from build123d import *

# Parameters (mm, degrees)
F0_W     = 76.2
F0_H     = 38.1
F1_DEPTH = 25.4
F2_R     = 3.175
F3_DEPTH = 25.4
F4_R     = 11.153796
F5_DEPTH = 38.1
F6_W     = 14.986
F6_H     = 12.7
F8_R     = 1.524


with BuildPart() as f1:
    # F0 (on Top) → F1 (new body)
    with BuildSketch(Plane.XY):
        with Locations((0.211801, -8.619163)):
            Rectangle(F0_W, F0_H)
    extrude(amount=F1_DEPTH)

    # F2 (on Top) → F3 (cut)
    with BuildSketch(Plane.XY):
        with Locations((-30.268199, 2.810837)):
            Circle(F2_R)
        with Locations((-30.268199, -20.049163)):
            Circle(F2_R)
        with Locations((30.691801, 2.810837)):
            Circle(F2_R)
        with Locations((30.691801, -20.049163)):
            Circle(F2_R)
    extrude(amount=F3_DEPTH, mode=Mode.SUBTRACT)

    # F4 (on face) → F5 (join)
    with BuildSketch(Plane.XY.offset(25.4)):
        with Locations((0, -7.839597)):
            Circle(F4_R)
    extrude(amount=F5_DEPTH)

    # F6 (on Front) → F7 (revolve, cut)
    with BuildSketch(Plane.XZ):
        with Locations((-11.421585, 44.041961)):
            Rectangle(F6_W, F6_H)
    revolve(axis=Axis((0, -7.839597, 63.5), (0, 0, 1)), mode=Mode.SUBTRACT)

    # F8
    f8_edges = [f1.edges().sort_by_distance(p)[0] for p in [
        (0.211801, -27.669163, 25.4),
        (-37.888199, -8.619163, 25.4),
        (0.211801, 10.430837, 25.4),
        (38.311801, -8.619163, 25.4),
    ]]
    fillet(f8_edges, radius=F8_R)


solid = f1.part
Check sheet for the modelled part. Datum: model origin and axes. Units: mm. A direction names the side the tool comes from. Coordinates: 2 decimals unless noted, no trailing zeros. Loops run counter-clockwise (first coordinate to the right, second up) from the corner with the lowest first, then second, coordinate; pieces in that order, holes last. Notation, with made-up numbers: (29, 61.25) -> (48, 61.25) arc R28 cw to (48, 94.25) -> close; hole circle Ø3 at (9.5, 89). An arc over 180 degrees is marked (long way). Write item = value, one per line. Start each with the question number.
1. Draft check along Z on faces 4 (the cylindrical face through (27.52, 2.95, 12.52)), 5 (the flat face through (0, -8, 0)), 6 (the flat face through (-2, 1, 37.692)). Enter one of: released by +Z, released by -Z, zero draft, split by the parting line, or undercut.
2. Section check C-C on x = 18.5. Record the cut outline in (y, z).
3. Tool access check on faces 1 (the cylindrical face through (5.147, -17.735, 56.854)), 2 (the flat face through (0, 10.431, 12)), 3 (the cylindrical face through (5.142, -0.737, 44.131)). Record the directions out of +Z, -Z, +X, -X, +Y, -Y that give a thin tool (end or side, any length) a straight path to the whole face; none if there is none.
4. Section check B-B on y = 7. Record the cut outline in (x, z).
5. Section check D-D on z = 5. Record the cut outline in (x, y) (3 decimals).
6. Material ranges on line 1 (Z direction, x = 30.5, y = -2.5); line 2 (X direction, y = -19, z = 22); line 3 (Y direction, x = -25, z = 24), recorded low to high.
7. Depth check by flat-ended pin: P1, Ø1.5, axis at x = -1.5, z = 32.5, coming from the +Y side; P2, Ø8.5, axis at x = -30.27, y = -20.05, coming from the +Z side; P3, Ø12, axis at y = -11, z = 47.5, coming from the -X side. Enter the tip coordinate at first touch or a pass-through.
8. Section check A-A on x = 29. Record the cut outline in (y, z), then the cut area to 3 significant figures.
Responses:
q1.face_4 = zero draft
q1.face_5 = released by -Z
q1.face_6 = undercut
q2.outline = (-27.67, 0) -> (10.43, 0) -> (10.43, 23.88) arc R1.52 ccw to (8.91, 25.4) -> (-26.15, 25.4) arc R1.52 ccw to (-27.67, 23.88) -> close
q3.face_1 = +Z
q3.face_2 = +Z, -Z, +X, -X, +Y
q3.face_3 = none
q4.outline = (-37.89, 0) -> (38.31, 0) -> (38.31, 23.88) arc R1.52 ccw to (36.79, 25.4) -> (-36.36, 25.4) arc R1.52 ccw to (-37.89, 23.88) -> close
q5.outline = (-37.888, -27.669) -> (38.312, -27.669) -> (38.312, 10.431) -> (-37.888, 10.431) -> close; hole circle Ø6.35 at (-30.268, -20.049); hole circle Ø6.35 at (-30.268, 2.811); hole circle Ø6.35 at (30.692, -20.049); hole circle Ø6.35 at (30.692, 2.811)
q6.line_1 = 0 to 25.4
q6.line_2 = -37.89 to -33.26, -27.27 to 27.7, 33.69 to 38.31
q6.line_3 = -27.66 to 10.43
q7.P1 = 3.29
q7.P2 = 25.4
q7.P3 = -11.15
q8.outline = (-27.67, 0) -> (-22.74, 0) -> (-22.74, 25.4) -> (-26.15, 25.4) arc R1.52 ccw to (-27.67, 23.88) -> close; (-17.36, 0) -> (0.12, 0) -> (0.12, 25.4) -> (-17.36, 25.4) -> close; (5.5, 0) -> (10.43, 0) -> (10.43, 23.88) arc R1.52 ccw to (8.91, 25.4) -> (5.5, 25.4) -> close
q8.area = 694 mm2
